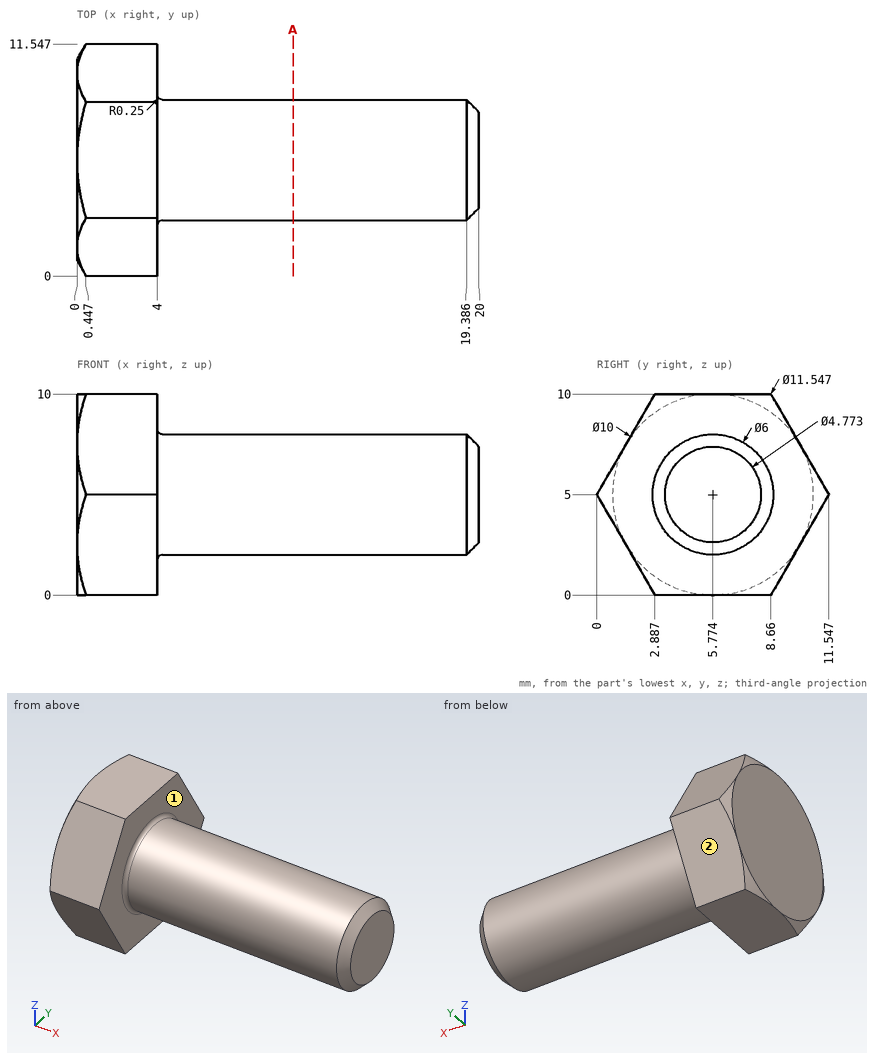
Geometry: see drawing. Coordinates: mm, zero at the bounding-box minimum. A direction names the side the tool comes from. Give positions to 0.01 mm unless a question says otherwise; leave off trailing zeros. Write each loop counter-clockwise with the first axis right and the second up, starting at its lowest first coordinate (ties: lowest second). Pieces come first, ordered by that corner, then holes. Notation, with made-up numbers: M 22.5,2.5 L 27.5,2.5 A37 cw 27.5,41.5 Z; hole C 38,61.25 d6. An arc over 180 degrees is marked long. Answer as a JSON object with one key per item and string values.
Q1. Cut plane A-A, the plane x = 10.75. Return the cut outline in (y, z).
Geometry check:
{"outline": "C 5.77,5 d6"}
Q2. Contact query for flat-ended pins moving along their axis: P1, Ø1.5, axis at y = 1.5, z = 3.5, coming from the +X side; P2, Ø5, axis at x = 15, z = 7, coming from the -Y side; P3, Ø5, axis at x = 12.5, y = 5.5, coming from the -Z side. Output: stop coordinate, or through.
Geometry check:
{"P1": "stops at x = 4", "P2": "stops at y = 2.77", "P3": "stops at z = 2"}
Q3. Access query for the marked faces 1 and 2. Directions: +Z, -Z, +X, -X, +Y, -Y. A direction counts if a zero-diameter tool reaches every point of the face in a straight line with its end or side. Return the directions, or none.
Geometry check:
{"face 1": "+X", "face 2": "-Z, +X, -X, +Y"}
Q4. Ray query, line 1 along X through (y, z) = (2.5, 8.5); line 2 along Z through (x, y) = (8, 7.75) (1 decimal); line 3 along Y through (x, z) = (3, 5.75) (1 decimal). Return the intervals inside material, ascending.
Geometry check:
{"line 1": "x = 0 to 4", "line 2": "z = 2.7 to 7.3", "line 3": "y = 0.4 to 11.1"}
